```python
from build123d import *

# Parameters (mm, degrees)
SKETCH1_R           = 6
SKETCH1_R_2         = 1.7
BOSS_EXTRUDE1_DEPTH = 3
SKETCH2_R           = 20
SKETCH2_R_2         = 6
SKETCH2_R_3         = 1.7
BOSS_EXTRUDE2_DEPTH = 2
SKETCH3_R           = 12
SKETCH3_R_2         = 6
BOSS_EXTRUDE3_DEPTH = 2
SKETCH4_R           = 6.5
SKETCH4_R_2         = 1.7
BOSS_EXTRUDE4_DEPTH = 2
SKETCH5_R           = 6.5
SKETCH5_R_2         = 1.7
BOSS_EXTRUDE5_DEPTH = 2
BOSS_EXTRUDE6_DEPTH = 0.6
SKETCH7_R           = 5.45
CUT_EXTRUDE1_DEPTH  = 0.6
SKETCH8_R           = 8.05
CUT_EXTRUDE2_DEPTH  = 4.5
SKETCH9_R           = 3.75
CUT_EXTRUDE3_DEPTH  = 2.3


with BuildPart() as part:
    # Sketch1 → Boss-Extrude1 (new body)
    with BuildSketch(Plane.XY.offset(328.5)):
        with BuildLine():
            Line((276.003127371, 300.387432585), (273.904807661, 170.421310226))
            ThreePointArc((273.904807661, 170.421310226), (300, 143.901406829), (326.095192339, 170.421310226))
            Line((326.095192339, 170.421310226), (323.996872629, 300.387432585))
            ThreePointArc((323.996872629, 300.387432585), (300, 324), (276.003127371, 300.387432585))
        make_face()
        with Locations((300, 300)):
            Circle(SKETCH1_R, mode=Mode.SUBTRACT)
        with Locations((300, 170)):
            Circle(SKETCH1_R, mode=Mode.SUBTRACT)
        with Locations((314.289419162, 308.25)):
            Circle(SKETCH1_R_2, mode=Mode.SUBTRACT)
        with Locations((285.710580838, 308.25)):
            Circle(SKETCH1_R_2, mode=Mode.SUBTRACT)
        with Locations((300, 240)):
            Circle(SKETCH1_R_2, mode=Mode.SUBTRACT)
        with Locations((300, 200)):
            Circle(SKETCH1_R_2, mode=Mode.SUBTRACT)
        with BuildLine():
            Line((305, 258.3), (314, 258.3))
            ThreePointArc((314, 258.3), (315.7, 260), (314, 261.7))
            Line((314, 261.7), (305, 261.7))
            ThreePointArc((305, 261.7), (303.3, 260), (305, 258.3))
        make_face(mode=Mode.SUBTRACT)
    extrude(amount=BOSS_EXTRUDE1_DEPTH)

    # Sketch2 → Boss-Extrude2 (add)
    with BuildSketch(Plane.XY.offset(331.5)):
        with Locations((300, 300)):
            Circle(SKETCH2_R)
        with Locations((300, 300)):
            Circle(SKETCH2_R_2, mode=Mode.SUBTRACT)
        with Locations((314.289419162, 308.25)):
            Circle(SKETCH2_R_3, mode=Mode.SUBTRACT)
        with Locations((285.710580838, 308.25)):
            Circle(SKETCH2_R_3, mode=Mode.SUBTRACT)
    extrude(amount=BOSS_EXTRUDE2_DEPTH)

    # Sketch3 → Boss-Extrude3 (add)
    with BuildSketch(Plane.XY.offset(331.5)):
        with Locations((300, 170)):
            Circle(SKETCH3_R)
        with Locations((300, 170)):
            Circle(SKETCH3_R_2, mode=Mode.SUBTRACT)
    extrude(amount=BOSS_EXTRUDE3_DEPTH)

    # Sketch4 → Boss-Extrude4 (add)
    with BuildSketch(Plane.XY.offset(331.5)):
        with Locations((300, 240)):
            Circle(SKETCH4_R)
        with Locations((300, 240)):
            Circle(SKETCH4_R_2, mode=Mode.SUBTRACT)
    extrude(amount=BOSS_EXTRUDE4_DEPTH)

    # Sketch5 → Boss-Extrude5 (add)
    with BuildSketch(Plane.XY.offset(331.5)):
        with Locations((300, 200)):
            Circle(SKETCH5_R)
        with Locations((300, 200)):
            Circle(SKETCH5_R_2, mode=Mode.SUBTRACT)
    extrude(amount=BOSS_EXTRUDE5_DEPTH)

    # Sketch6 → Boss-Extrude6 (add)
    with BuildSketch(Plane.XY.offset(333.5)):
        with BuildLine():
            Line((282.710827179, 300.61196663), (278.11511203, 170.774636315))
            ThreePointArc((278.11511203, 170.774636315), (300, 148.101406829), (321.88488797, 170.774636315))
            Line((321.88488797, 170.774636315), (317.289172821, 300.61196663))
            ThreePointArc((317.289172821, 300.61196663), (300, 317.3), (282.710827179, 300.61196663))
        make_face()
        with BuildLine():
            Line((283.910076161, 300.569518077), (279.314361012, 170.732187763))
            ThreePointArc((279.314361012, 170.732187763), (300, 149.301406829), (320.685638988, 170.732187763))
            Line((320.685638988, 170.732187763), (316.089923839, 300.569518077))
            ThreePointArc((316.089923839, 300.569518077), (300, 316.1), (283.910076161, 300.569518077))
        make_face(mode=Mode.SUBTRACT)
    extrude(amount=BOSS_EXTRUDE6_DEPTH)

    # Sketch7 → Cut-Extrude1 (cut)
    with BuildSketch(Plane.XY.offset(333.5)):
        with Locations((314.289419162, 308.25)):
            Circle(SKETCH7_R)
        with Locations((285.710580838, 308.25)):
            Circle(SKETCH7_R)
    extrude(amount=CUT_EXTRUDE1_DEPTH, mode=Mode.SUBTRACT)

    # Sketch8 → Cut-Extrude2 (cut)
    with BuildSketch(Plane.XY.offset(329)):
        with Locations((300, 300)):
            Circle(SKETCH8_R)
        with Locations((300, 170)):
            Circle(SKETCH8_R)
    extrude(amount=CUT_EXTRUDE2_DEPTH, mode=Mode.SUBTRACT)

    # Sketch9 → Cut-Extrude3 (cut)
    with BuildSketch(Plane.XY.offset(328.5)):
        with Locations((314.289419162, 308.25)):
            Circle(SKETCH9_R)
        with Locations((285.710580838, 308.25)):
            Circle(SKETCH9_R)
        with Locations((300, 240)):
            Circle(SKETCH9_R)
        with Locations((300, 200)):
            Circle(SKETCH9_R)
    extrude(amount=CUT_EXTRUDE3_DEPTH, mode=Mode.SUBTRACT)


solid = part.part
```
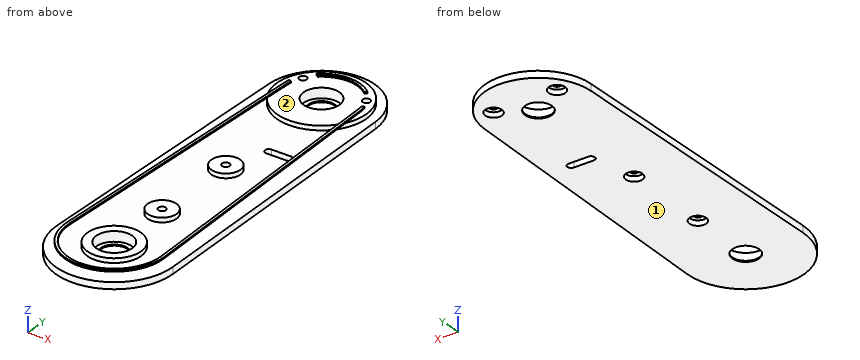
Here's how the part is built. I have some questions about the finished solid (model axes, mm). Face numbers are marked on the shaded views. Give positions to 0.01 mm unless a question says otherwise; leave off trailing zeros. Order: outer loops, then holes, each group sorted by start corner. A loop starts at its lowest first (then second) coordinate and runs counter-clockwise, first axis right, second up. Notation, with made-up numbers: (64, 68.25) -> (93, 68.25) arc R20 ccw to (93, 104.25) -> close; hole circle Ø1 at (4, 4.25). An arc over 180 degrees is marked (long way). Use CSV: the item, a comma, the result in double quotes. Start each with the question number.
Item 1: Suppose I cut it at A-A (y = 186). List the corners of the cut face in (x, z) for me.
Item 2: Suppose I cut it at B-B (x = 300). Give the number of separate pieces and of enclosed holes in the cut face, and give its area (3 significant figures).
Item 3: Suppose I cut it at D-D (y = 216). List the corners of the cut face in (x, z) for me, and give its area (3 significant figures).
Item 4: I'm going to push flat-ended pins straight in: P1, Ø3, axis at x = 304, z = 331, coming from the -Y side; P2, Ø4, axis at x = 299, y = 240.5, coming from the +Z side; P3, Ø5, axis at x = 298.5, y = 173.5, coming from the +Z side. Where does each tip first touch, or does it pass through?
Item 5: Suppose I cut it at C-C (y = 240). List the corners of the cut face in (x, z) for me, and give its area (3 significant figures).
Item 6: If I drill on probe 1 along Y at (x, z) = (296.5, 332.6); probe 2 along X at (y, z) = (300, 328.95); probe 3 along Y at (x, z) = (297, 331.3), over which ranges is the centre line in solid material (lowest first)? Write a range as [from, to].
Item 7: Thinking about a two-plate mould opening in Y: for the marked faces 1 and 2, which applies, pulls with the +Y half, pulls with the -Y half, needs draft (parallel to the pull), parting line crosses it, or undercut?
Answer block:
1,outline,"(274.16, 328.5) -> (325.84, 328.5) -> (325.84, 331.5) -> (274.16, 331.5) -> close; (278.65, 333.5) -> (279.85, 333.5) -> (279.85, 334.1) -> (278.65, 334.1) -> close; (320.15, 333.5) -> (321.35, 333.5) -> (321.35, 334.1) -> (320.15, 334.1) -> close"
2,separate pieces,"6"
2,enclosed holes,"0"
2,area,"512 mm^2"
3,outline,"(274.64, 328.5) -> (325.36, 328.5) -> (325.36, 331.5) -> (274.64, 331.5) -> close; (279.72, 333.5) -> (280.92, 333.5) -> (280.92, 334.1) -> (279.72, 334.1) -> close; (319.08, 333.5) -> (320.28, 333.5) -> (320.28, 334.1) -> (319.08, 334.1) -> close"
3,area,"154 mm^2"
4,P1,"stops at y = 144.02"
4,P2,"stops at z = 333.5"
4,P3,"stops at z = 329"
5,outline,"(275.03, 328.5) -> (296.25, 328.5) -> (296.25, 330.8) -> (298.3, 330.8) -> (298.3, 333.5) -> (293.5, 333.5) -> (293.5, 331.5) -> (275.03, 331.5) -> close; (280.57, 333.5) -> (281.77, 333.5) -> (281.77, 334.1) -> (280.57, 334.1) -> close; (301.7, 330.8) -> (303.75, 330.8) -> (303.75, 328.5) -> (324.97, 328.5) -> (324.97, 331.5) -> (306.5, 331.5) -> (306.5, 333.5) -> (301.7, 333.5) -> close; (318.23, 333.5) -> (319.43, 333.5) -> (319.43, 334.1) -> (318.23, 334.1) -> close"
5,area,"151 mm^2"
6,probe 1,"y = [158.52, 162.75], [177.25, 181.48], [194.52, 205.48], [234.52, 245.48], [280.31, 292.75], [307.25, 319.69]"
6,probe 2,"x = [276, 294], [306, 324]"
6,probe 3,"y = [144.07, 162.53], [177.47, 292.53], [307.47, 323.81]"
7,face 1,"needs draft"
7,face 2,"undercut"
